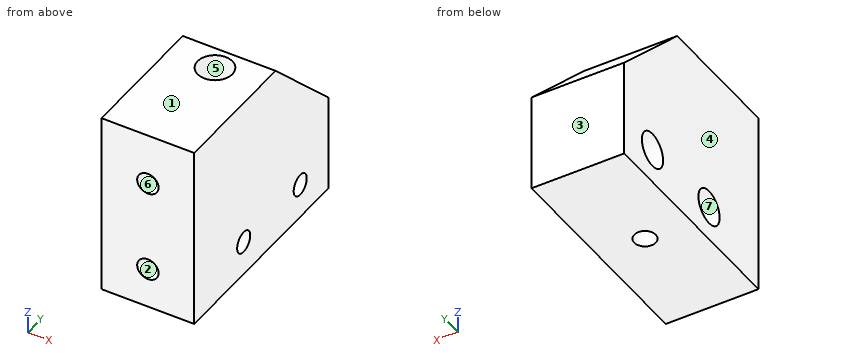
Autodesk Inventor part; units mm, degrees
ref_plane "YZ Plane" through (0, 0, 0) normal (1, 0, 0) x (0, 1, 0)
ref_plane "XZ Plane" through (0, 0, 0) normal (0, 1, 0) x (-1, 0, 0)
ref_plane "XY Plane" through (0, 0, 0) normal (0, 0, 1) x (1, 0, 0)
sketch "Sketch1" plane through (0, 0, 0) normal (0, 1, 0) x (-1, 0, 0)
  line L0 (0, 0) -> (16, 0)
  line L1 (16, 0) -> (16, -32)
  line L2 (16, -32) -> (0, -32)
  line L3 (0, -32) -> (0, 0)
  dimension "d0" = 16
  dimension "d1" = 32
extrude "Extrusion1" add sketch "Sketch1" along normal blind 38
sketch "Sketch2" plane through (-16, 0, -32) normal (-1, 0, 0) x (0, 0, 1)
  circle A0 centre (6, 14) radius 1.3525
  circle A1 centre (6, 30) radius 1.3525
  point P0 (32, 0)
hole "Hole1" at (-16, 14, -26) at (-16, 30, -26) direction (1, 0, 0) diameter 3.7 end through all counterbore diameter 6 counterbore depth 10
sketch "Sketch3" plane through (0, 0, 0) normal (0, -1, 0) x (1, 0, 0)
  circle A0 centre (-8, -25) radius 1.85
  circle A1 centre (-8, -9) radius 1.85
  point P0 (0, 0)
hole "Hole2" at (-8, 0, -25) at (-8, 0, -9) direction (0, 1, 0) diameter 3.7 depth 8
chamfer "Chamfer1" distance 15 angle 45 1 edges at (-8, 38, 0)
sketch "Sketch4" plane through (0, 0, -32) normal (0, 0, -1) x (-1, 0, 0)
  line L0 (0, 0) -> (16, 0)
  line L1 (16, 0) -> (16, 38)
  line L2 (0, 38) -> (16, 38)
  line L3 (0, 0) -> (0, 38)
  point P0 (8, 19)
hole "Hole3" at (-8, 19, -32) direction (0, 0, 1) diameter 3.7 end through all
sketch "Sketch6" plane through (-16, 0, 0) normal (0, 0, 1) x (1, 0, 0)
  circle A0 centre (8, 19) radius 1.85
  point P0 (16, 0)
hole "Hole5" at (-8, 19, 0) direction (0, 0, -1) diameter 6 depth 10
properties part number "innerbracket" material "ABS Plastic"
Geometry: final body of the model. Coordinates: model frame, mm. Face numbers are marked on the shaded views. A direction names the side the tool comes from. Give positions to 0.01 mm unless a question says otherwise; leave off trailing zeros. Write each loop counter-clockwise with the first axis right and the second up, starting at its lowest first coordinate (ties: lowest second). Pieces come first, ordered by that corner, then holes. Notation, with made-up numbers: (49, -17) -> (102, -17) arc R23 cw to (102, 11) -> close; hole circle Ø9 at (-20.75, 36). An arc over 180 degrees is marked (long way). Answer as a JSON object with one key per item and string values.
1. Cut plane A-A on x = -8. Output: boundary loops of the cut face in (y, z), and give its area (3 significant figures).
Ans:
{"outline": "(0, -32) -> (17.15, -32) -> (17.15, -10) -> (16, -10) -> (16, 0) -> (0, 0) -> (0, -7.15) -> (8, -7.15) -> (8, -10.85) -> (0, -10.85) -> (0, -23.15) -> (8, -23.15) -> (8, -26.85) -> (0, -26.85) -> close; (20.85, -32) -> (38, -32) -> (38, -15) -> (23, 0) -> (22, 0) -> (22, -10) -> (20.85, -10) -> close; hole circle Ø6 at (14, -26); hole circle Ø6 at (30, -26)", "area": "846 mm^2"}
2. Cut plane B-B on z = -25.5. Output: boundary loops of the cut face in (x, y), and give its area (3 significant figures).
Ans:
{"outline": "(-16, 0) -> (-9.78, 0) -> (-9.78, 8) -> (-6.22, 8) -> (-6.22, 0) -> (0, 0) -> (0, 12.22) -> (-6, 12.22) -> (-6, 11.04) -> (-16, 11.04) -> close; (-16, 16.96) -> (-6, 16.96) -> (-6, 15.78) -> (0, 15.78) -> (0, 28.22) -> (-6, 28.22) -> (-6, 27.04) -> (-16, 27.04) -> close; (-16, 32.96) -> (-6, 32.96) -> (-6, 31.78) -> (0, 31.78) -> (0, 38) -> (-16, 38) -> close; hole circle Ø3.7 at (-8, 19)", "area": "408 mm^2"}
3. Contact query for flat-ended pins moving along their axis: pin 1 (4.5 mm diameter, centred on x = -8, z = -9, fed in from -Y); pin 2 (1.8 mm diameter, centred on y = 12.5, z = -25, fed in from -X); pin 3 (1.1 mm diameter, centred on x = -7.5, z = -8.5, fed in from -Y); pin 4 (1.8 mm diameter, centred on x = -7, y = 18.5, fed in from +Z). Output: stop coordinate, or through.
Ans:
{"pin 1": "stops at y = 0", "pin 2": "stops at x = -6", "pin 3": "stops at y = 8", "pin 4": "stops at z = -10"}
4. Access query for the marked faces 4, 5, 6 and 7. Directions: +Z, -Z, +X, -X, +Y, -Y. A direction counts if a zero-diameter tool reaches every point of the face in a straight line with its end or side. Return the directions, or none.
Ans:
{"face 4": "+Z, -Z, -X, +Y, -Y", "face 5": "+Z", "face 6": "-Y", "face 7": "-X"}
5. Mould query, pull axis Z, two halves, no side actions, for the marked faces 1, 2 and 3. Classes: pulls with the +Z half, pulls with the -Z half, needs draft (parallel to the pull), parting line crosses it, or undercut.
Ans:
{"face 1": "pulls with the +Z half", "face 2": "undercut", "face 3": "needs draft"}
6. Cut plane C-C on y = 14. Output: boundary loops of the cut face in (x, z), and give its area (3 significant figures).
Ans:
{"outline": "(-16, -32) -> (0, -32) -> (0, -27.85) -> (-6, -27.85) -> (-6, -29) -> (-16, -29) -> close; (-16, -23) -> (-6, -23) -> (-6, -24.15) -> (0, -24.15) -> (0, 0) -> (-16, 0) -> close", "area": "430 mm^2"}
7. Cut plane D-D on x = -4.25. Output: boundary loops of the cut face in (y, z).
Ans:
{"outline": "(0, -32) -> (38, -32) -> (38, -15) -> (23, 0) -> (0, 0) -> close; hole circle Ø3.7 at (14, -26); hole circle Ø3.7 at (30, -26)"}
8. Ray query, probe 1 along Y at (x, z) = (-2.05, -26); probe 2 along Y at (x, z) = (-13.5, -26); probe 3 along Z at (x, y) = (-8.75, 2). Return the intervals inside material, ascending. Write a range as from..to.
Ans:
{"probe 1": "y = 0..12.15, 15.85..28.15, 31.85..38", "probe 2": "y = 0..11, 17..27, 33..38", "probe 3": "z = -32..-26.69, -23.31..-10.69, -7.31..0"}
